Geometry check sheet. Reference: the model listing, model coordinates, mm. A direction names the side the tool comes from. Give positions to 0.01 mm unless a question says otherwise; leave off trailing zeros. Order: outer loops, then holes, each group sorted by start corner. A loop starts at its lowest first (then second) coordinate and runs counter-clockwise, first axis right, second up.
```python
from build123d import *

# Parameters (mm, degrees)
SKETCH1_W                = 97
SKETCH1_H                = 19
BOSS_EXTRUDE1_DEPTH      = 10
SKETCH4_W                = 19.5
SKETCH4_H                = 19
CUT_EXTRUDE1_DEPTH       = 5
BOSS_EXTRUDE2_DEPTH      = 45.5
BOSS_EXTRUDE2_DEPTH_BACK = 29.5
SKETCH6_W                = 26.3
SKETCH6_H                = 19
SKETCH6_W_2              = 45.2
CUT_EXTRUDE2_DEPTH       = 2
SKETCH7_W                = 29.3
SKETCH7_H                = 19
SKETCH7_W_2              = 48.2
CUT_EXTRUDE3_DEPTH       = 1


with BuildPart() as part:
    # Sketch1 → Boss-Extrude1 (new body)
    with BuildSketch(Plane(origin=(0, 0, 0), x_dir=(1, 0, 0), z_dir=(0, 1, 0))):
        Rectangle(SKETCH1_W, SKETCH1_H)
    extrude(amount=-BOSS_EXTRUDE1_DEPTH)

    # Sketch4 → Cut-Extrude1 (cut)
    with BuildSketch(Plane(origin=(0, 0, 0), x_dir=(1, 0, 0), z_dir=(0, 1, 0))):
        with Locations((-9.45, 0)):
            Rectangle(SKETCH4_W, SKETCH4_H)
    extrude(amount=-CUT_EXTRUDE1_DEPTH, mode=Mode.SUBTRACT)

    # Sketch5 → Boss-Extrude2 (add, two sides: drawn at the far end of the back side and taken through both)
    with BuildSketch(Plane.ZY.offset(-0.3).offset(-BOSS_EXTRUDE2_DEPTH_BACK)):
        Polygon((-2.5, -5), (0, 2), (2.5, -5), align=None)
    extrude(amount=BOSS_EXTRUDE2_DEPTH + BOSS_EXTRUDE2_DEPTH_BACK)

    # Sketch6 → Cut-Extrude2 (cut)
    with BuildSketch(Plane(origin=(0, 0, 0), x_dir=(1, 0, 0), z_dir=(0, 1, 0))):
        with Locations((-32.35, 0)):
            Rectangle(SKETCH6_W, SKETCH6_H)
        with Locations((22.9, 0)):
            Rectangle(SKETCH6_W_2, SKETCH6_H)
    extrude(amount=CUT_EXTRUDE2_DEPTH, mode=Mode.SUBTRACT)

    # Sketch7 → Cut-Extrude3 (cut)
    with BuildSketch(Plane(origin=(0, 0, 0), x_dir=(1, 0, 0), z_dir=(0, 1, 0))):
        with Locations((-33.85, 0)):
            Rectangle(SKETCH7_W, SKETCH7_H)
        with Locations((24.4, 0)):
            Rectangle(SKETCH7_W_2, SKETCH7_H)
    extrude(amount=-CUT_EXTRUDE3_DEPTH, mode=Mode.SUBTRACT)


solid = part.part
```
Q1. Release check for a two-part mould opening along X. For faces 1 (the face through (-9.314, -1.451, 1.232)), 2 (the face through (0.3, 0, 0)), 3 (the face through (-0.7, -5.4, -9.5)), 4 (the face through (0.3, -3, -5)) record: pulls with the +X half, pulls with the -X half, needs draft (parallel to the pull), parting line crosses it, or undercut.
Q2. Cross-section at C-C, the plane y = 0.75. Record the boundary of the cut face in (x, z), and give its area (3 significant figures).
Q3. Cross-section at D-D, the plane x = -29. Record the boundary of the cut face in (y, z), and give its area (3 significant figures).
Q4. Cross-section at A-A, the plane x = -8.5. Record the boundary of the cut face in (y, z).
Q5. Cross-section at B-B, the plane z = 7.5. Record the boundary of the cut face in (x, y), and give its area (3 significant figures).
Q6. Access from +Z, -Z, +X, -X, +Y, -Y to the whole of each face (thin tool, end or side, straight path). Record for faces 5 (the face through (-9.314, -1.549, -1.268)), 6 (the face through (-19.2, 0, 0)), 7 (the face through (-19.2, -3, 5)).
Q7. Gauge pin test, flat ends, axial feed: P1, Ø3.5, axis at x = -10.5, z = 5.5, coming from the +Y side; P2, Ø5.5, axis at x = 30, z = -4, coming from the +Y side; P3, Ø1.1, axis at y = 1, z = 0.5, coming from the +X side. Record the tip position at first contact, or that the pin passes through.
Q8. Thickness scan on L1, parallel to X at y = -3.5, z = 4.75; L2, parallel to Y at x = 18.5, z = -7.75; L3, parallel to Y at x = -19, z = 5.75. Record the ranges inside material, lowest first.
Answers follow:
1. face 1: undercut
1. face 2: pulls with the +X half
1. face 3: needs draft
1. face 4: undercut
2. outline: (-19.2, -0.45) - (0.3, -0.45) - (0.3, 0.45) - (-19.2, 0.45) - close
2. area: 17.4 mm2
3. outline: (-10, -9.5) - (-1, -9.5) - (-1, 9.5) - (-10, 9.5) - close
3. area: 171 mm2
4. outline: (-10, -9.5) - (-5, -9.5) - (-5, -2.5) - (2, 0) - (-5, 2.5) - (-5, 9.5) - (-10, 9.5) - close
5. outline: (-48.5, -10) - (48.5, -10) - (48.5, -1) - (0.3, -1) - (0.3, -5) - (-19.2, -5) - (-19.2, -1) - (-48.5, -1) - close
5. area: 795 mm2
6. face 5: -Z, +Y
6. face 6: +Z, -Z, -X, +Y
6. face 7: +Z, +Y
7. P1: stops at y = -5
7. P2: stops at y = -1
7. P3: stops at x = 0.3
8. L1: x = -48.5 to -19.2, 0.3 to 48.5
8. L2: y = -10 to -1
8. L3: y = -10 to -5
